```python
from build123d import *

# Parameters (mm, degrees)
F1_DEPTH  = 50.8
F3_DEPTH  = 76.2
F4_R      = 38.1
F1_FACE_R = 12.7
F5_DEPTH  = 12.7


with BuildPart() as f1:
    # F0 (on Front) → F1 (new body, symmetric)
    with BuildSketch(Plane.XZ):
        with BuildLine():
            ThreePointArc((-130.8751894546, 96.1189323328), (-190.1214960247, 111.9939323328), (-146.7501894546, 68.6226257627))
            Line((-146.7501894546, 68.6226257627), (-156.2751894546, 85.1204097048))
            ThreePointArc((-156.2751894546, 85.1204097048), (-173.6237120826, 102.4689323328), (-149.9251894546, 96.1189323328))
            Line((-149.9251894546, 96.1189323328), (-130.8751894546, 96.1189323328))
        make_face()
        with BuildLine():
            Line((-156.2751894546, 85.1204097048), (-146.7501894546, 68.6226257627))
            ThreePointArc((-146.7501894546, 68.6226257627), (-135.1288828844, 80.2439323328), (-130.8751894546, 96.1189323328))
            Line((-130.8751894546, 96.1189323328), (-149.9251894546, 96.1189323328))
            ThreePointArc((-149.9251894546, 96.1189323328), (-151.6266668265, 89.7689323328), (-156.2751894546, 85.1204097048))
        make_face()
        with BuildLine():
            Line((181.3982178505, 85.1204097048), (171.8732178505, 68.6226257627))
            ThreePointArc((171.8732178505, 68.6226257627), (203.6232178505, 68.6226257627), (219.4982178505, 96.1189323328))
            ThreePointArc((219.4982178505, 96.1189323328), (187.7482178505, 127.8689323328), (155.9982178505, 96.1189323328))
            Line((155.9982178505, 96.1189323328), (175.0482178505, 96.1189323328))
            ThreePointArc((175.0482178505, 96.1189323328), (187.7482178505, 108.8189323328), (200.4482178505, 96.1189323328))
            ThreePointArc((200.4482178505, 96.1189323328), (194.0982178505, 85.1204097048), (181.3982178505, 85.1204097048))
        make_face()
        with BuildLine():
            ThreePointArc((-79.513485802, -47.834761097), (-47.763485802, -47.834761097), (-31.888485802, -75.3310676672))
            Line((-31.888485802, -75.3310676672), (57.011514198, -75.3310676672))
            ThreePointArc((57.011514198, -75.3310676672), (72.886514198, -47.834761097), (104.636514198, -47.834761097))
            Line((104.636514198, -47.834761097), (171.8732178505, 68.6226257627))
            ThreePointArc((171.8732178505, 68.6226257627), (160.2519112804, 80.2439323328), (155.9982178505, 96.1189323328))
            Line((155.9982178505, 96.1189323328), (-130.8751894546, 96.1189323328))
            ThreePointArc((-130.8751894546, 96.1189323328), (-135.1288828844, 80.2439323328), (-146.7501894546, 68.6226257627))
            Line((-146.7501894546, 68.6226257627), (-79.513485802, -47.834761097))
        make_face()
        with BuildLine():
            Line((76.061514198, -75.3310676672), (57.011514198, -75.3310676672))
            ThreePointArc((57.011514198, -75.3310676672), (88.761514198, -107.0810676672), (120.511514198, -75.3310676672))
            ThreePointArc((120.511514198, -75.3310676672), (116.2578207681, -59.4560676672), (104.636514198, -47.834761097))
            Line((104.636514198, -47.834761097), (95.111514198, -64.3325450391))
            ThreePointArc((95.111514198, -64.3325450391), (99.760036826, -68.9810676672), (101.461514198, -75.3310676672))
            ThreePointArc((101.461514198, -75.3310676672), (88.761514198, -88.0310676672), (76.061514198, -75.3310676672))
        make_face()
        with BuildLine():
            ThreePointArc((104.636514198, -47.834761097), (72.886514198, -47.834761097), (57.011514198, -75.3310676672))
            Line((57.011514198, -75.3310676672), (76.061514198, -75.3310676672))
            ThreePointArc((76.061514198, -75.3310676672), (82.411514198, -64.3325450391), (95.111514198, -64.3325450391))
            Line((95.111514198, -64.3325450391), (104.636514198, -47.834761097))
        make_face()
        with BuildLine():
            Line((-31.888485802, -75.3310676672), (-50.938485802, -75.3310676672))
            ThreePointArc((-50.938485802, -75.3310676672), (-69.988485802, -86.3295902952), (-69.988485802, -64.3325450391))
            Line((-69.988485802, -64.3325450391), (-79.513485802, -47.834761097))
            ThreePointArc((-79.513485802, -47.834761097), (-79.513485802, -102.8273742373), (-31.888485802, -75.3310676672))
        make_face()
        with BuildLine():
            ThreePointArc((-69.988485802, -64.3325450391), (-57.288485802, -64.3325450391), (-50.938485802, -75.3310676672))
            Line((-50.938485802, -75.3310676672), (-31.888485802, -75.3310676672))
            ThreePointArc((-31.888485802, -75.3310676672), (-47.763485802, -47.834761097), (-79.513485802, -47.834761097))
            Line((-79.513485802, -47.834761097), (-69.988485802, -64.3325450391))
        make_face()
        with BuildLine():
            ThreePointArc((155.9982178505, 96.1189323328), (160.2519112804, 80.2439323328), (171.8732178505, 68.6226257627))
            Line((171.8732178505, 68.6226257627), (181.3982178505, 85.1204097048))
            ThreePointArc((181.3982178505, 85.1204097048), (176.7496952225, 89.7689323328), (175.0482178505, 96.1189323328))
            Line((175.0482178505, 96.1189323328), (155.9982178505, 96.1189323328))
        make_face()
    extrude(amount=F1_DEPTH, both=True)

    # F2 (on face) → F3 (cut)
    with BuildSketch(Plane.XZ.offset(50.8)):
        Polygon((136.4217789196, 96.1189323328), (-111.2987505236, 96.1189323328), (-32.3154252183, -40.6842000468), (57.4384536142, -40.6842000468), align=None)
    extrude(amount=-F3_DEPTH, mode=Mode.SUBTRACT)

    # F4 (on Front) + F1_face (on face) → F5 (cut, symmetric)
    with BuildSketch(Plane.XZ):
        with Locations((-162.6251894546, 96.1189323328)):
            Circle(F4_R)
    with BuildSketch(Plane(origin=(12.561514198, -50.8, 21.3503423812), x_dir=(1, 0, 0), z_dir=(0, -1, 0))):
        with BuildLine():
            Line((-123.8602647216, 74.7685899517), (-143.4367036526, 74.7685899517))
            ThreePointArc((-143.4367036526, 74.7685899517), (-202.6830102227, 90.6435899517), (-159.3117036526, 47.2722833815))
            Line((-159.3117036526, 47.2722833815), (-92.075, -69.1851034782))
            ThreePointArc((-92.075, -69.1851034782), (-92.075, -124.1777166185), (-44.45, -96.6814100483))
            Line((-44.45, -96.6814100483), (44.45, -96.6814100483))
            ThreePointArc((44.45, -96.6814100483), (92.075, -124.1777166185), (92.075, -69.1851034782))
            Line((92.075, -69.1851034782), (159.3117036526, 47.2722833815))
            ThreePointArc((159.3117036526, 47.2722833815), (202.6830102227, 90.6435899517), (143.4367036526, 74.7685899517))
            Line((143.4367036526, 74.7685899517), (123.8602647216, 74.7685899517))
            Line((123.8602647216, 74.7685899517), (44.8769394163, -62.0345424279))
            Line((44.8769394163, -62.0345424279), (-44.8769394163, -62.0345424279))
            Line((-44.8769394163, -62.0345424279), (-123.8602647216, 74.7685899517))
        make_face()
        with Locations((-76.2, -96.6814100483)):
            Circle(F1_FACE_R, mode=Mode.SUBTRACT)
        with Locations((76.2, -96.6814100483)):
            Circle(F1_FACE_R, mode=Mode.SUBTRACT)
        with Locations((-175.1867036526, 74.7685899517)):
            Circle(F1_FACE_R, mode=Mode.SUBTRACT)
        with Locations((175.1867036526, 74.7685899517)):
            Circle(F1_FACE_R, mode=Mode.SUBTRACT)
    extrude(amount=F5_DEPTH, both=True, mode=Mode.SUBTRACT)


solid = f1.part
```
Geometry check sheet. Reference: the model listing, model coordinates, mm. A direction names the side the tool comes from. Coordinates: 2 decimals unless noted, no trailing zeros. Loops run counter-clockwise (first coordinate to the right, second up) from the corner with the lowest first, then second, coordinate; pieces in that order, holes last. Notation, with made-up numbers: (46.25, -25.75) - (75.25, -25.75) arc R6 ccw to (75.25, -14.75) - close; hole circle Ø8 at (-14, -2.75). An arc over 180 degrees is marked (long way). One line per item, written item: value. Start each with the question number.
(1) Cross-section at C-C on y = -4. Enter the section's corners in (x, z).
(2) Cross-section at D-D on x = -6.5. Enter the section's corners in (y, z).
(3) Mould release check, pull along Y, two halves, no side actions. Record for faces 1 (the flat face through (15, 35, 96.119)), 2 (the flat face through (-160, 12.7, 82)), 3 (the flat face through (10, 50.8, 12)): released by +Y, released by -Y, zero draft, split by the parting line, or undercut.
(4) Depth check by flat-ended pin: P1, Ø5, axis at x = -12.5, y = 23, coming from the +Z side; P2, Ø8, axis at x = 60.5, y = 27, coming from the -Z side; P3, Ø10, axis at x = 106, y = -7.5, coming from the -Z side; P4, Ø23, axis at x = -162.63, z = 96.12, coming from the +Y side. Enter the tip coordinate at first touch or a pass-through.
(5) Cross-section at A-A on y = 18. Enter the section's corners in (x, z), plus the area to 3 significant figures.
(6) Material ranges on line 1 (X direction, y = 12.5, z = -75); line 2 (X direction, y = 6, z = 88); line 3 (Y direction, x = 11, z = -7), recorded low to high. Write a range as [from, to].
(7) Tool access check on faces 4 (the flat face through (-160, -12.7, 82)), 5 (the flat face through (12, 6, -75.331)), 6 (the cylindrical face through (215.808, 5.728, 110.976)), 7 (the flat face through (12, -7, -40.684)). Record the directions out of +Z, -Z, +X, -X, +Y, -Y that give a thin tool (end or side, any length) a straight path to the whole face; none if there is none.
(8) Cross-section at B-B on z = -79.5. Enter the section's corners in (x, y), plus the area to 3 significant figures.
Results below:
1. outline: (-143.58, 63.12) - (-79.51, -47.83) arc R31.75 ccw (long way) to (-31.89, -75.33) - (57.01, -75.33) arc R31.75 ccw (long way) to (104.64, -47.83) - (171.87, 68.62) arc R31.75 ccw (long way) to (156, 96.12) - (136.42, 96.12) - (57.44, -40.68) - (-32.32, -40.68) - (-111.3, 96.12) - (-124.53, 96.12) arc R38.1 cw to start; hole circle Ø25.4 at (-63.64, -75.33); hole circle Ø25.4 at (88.76, -75.33); hole circle Ø25.4 at (187.75, 96.12)
2. outline: (-38.1, -75.33) - (50.8, -75.33) - (50.8, 96.12) - (25.4, 96.12) - (25.4, -40.68) - (-38.1, -40.68) - close
3. face 1: zero draft
3. face 2: undercut
3. face 3: released by +Y
4. P1: stops at z = 96.12
4. P2: stops at z = -95.81
4. P3: stops at z = -104.63
4. P4: passes through
5. outline: (-146.75, 68.62) - (-79.51, -47.83) arc R31.75 ccw (long way) to (-31.89, -75.33) - (57.01, -75.33) arc R31.75 ccw (long way) to (104.64, -47.83) - (171.87, 68.62) arc R31.75 ccw (long way) to (156, 96.12) - (136.42, 96.12) - (57.44, -40.68) - (-32.32, -40.68) - (-111.3, 96.12) - (-130.88, 96.12) arc R31.75 ccw (long way) to start; hole circle Ø25.4 at (-162.63, 96.12); hole circle Ø25.4 at (-63.64, -75.33); hole circle Ø25.4 at (88.76, -75.33); hole circle Ø25.4 at (187.75, 96.12)
5. area: 27,500 mm2
6. line 1: x = [-95.39, -76.33], [-50.94, 76.07], [101.46, 120.51]
6. line 2: x = [-125.4, -106.61], [131.73, 177.98], [197.51, 218.44]
6. line 3: y = [25.4, 50.8]
7. face 4: +Z, -X
7. face 5: -Z, +Y, -Y
7. face 6: +Y, -Y
7. face 7: +Z, -Y
8. outline: (-95.11, -38.1) - (-75.63, -38.1) - (-75.63, 50.8) - (-95.11, 50.8) - close; (-51.64, -38.1) - (-32.16, -38.1) - (-32.16, 50.8) - (-51.64, 50.8) - close; (57.29, -38.1) - (76.77, -38.1) - (76.77, 50.8) - (57.29, 50.8) - close; (100.76, -38.1) - (120.24, -38.1) - (120.24, 50.8) - (100.76, 50.8) - close
8. area: 6,930 mm2
